Model file for the job. Use its own axes, mm. A direction names the side the tool comes from. Coordinates: 2 decimals unless noted, no trailing zeros. Order: outer loops, then holes, each group sorted by start corner. A loop starts at its lowest first (then second) coordinate and runs counter-clockwise, first axis right, second up. Notation, with made-up numbers: (19, 87.5) -> (45, 87.5) arc R20 cw to (45, 106.5) -> close; hole circle Ø3 at (79, 74.5). An arc over 180 degrees is marked (long way). Use CSV: the item, a comma, the result in double quotes. Start each with the question number.
(1) Cut at A-A on x = 18. Write the cut outline in (y, z), plus the area to 3 significant figures.
(2) Cut at B-B on y = 58.25. Write the cut outline in (x, z).
(3) Probe L1, parallel to Y at x = 18, z = 0.65; L2, parallel to X at y = 58, z = 2.05; L3, parallel to X at y = 43, z = 2.05. List the from-to ranges inside material, lowest first.
(4) Tool access for faces 4 (the flat face through (-22, 55, 1)), 5 (the flat face through (38, 33, 1)), 6 (the flat face through (1, 0, 1)): list every direction of +Z, -Z, +X, -X, +Y, -Y with a clear straight run to the whole face (end or side of a thin tool).
(5) Cut at D-D on x = -26. Write the cut outline in (y, z).
(6) Pin check, flat tips, straight feed: pin 1 Ø3 at (x, y) = (-18, 41.75) entering from -Z (3 decimals); pin 2 Ø1.5 at (x, z) = (38, 2) entering from +Y; pin 3 Ø1.5 at (y, z) = (58.5, 1) entering from +X. Stop position of each tip, or through.
(7) Cut at C-C on z = 2.4. Give the number of separate pieces and of enclosed holes in the cut face, plus the area to 3 significant figures.
(8) Pull direction Y, two halves, no side cores. Call faces 1 (the flat face through (40, 17, 1)), 2 (the cylindrical face through (26.51, 37.28, 1.52)), 3 (the cylindrical face through (17.566, 39.798, 1.521)): pulls with the +Y half, pulls with the -Y half, needs draft (parallel to the pull), parting line crosses it, or undercut.
```python
from build123d import *

# Parameters (mm, degrees)
EXTRUDE_1_DEPTH     = 3
SKETCH_2_R          = 2
CUT_EXTRUDE_1_DEPTH = 75.054456314
SKETCH_3_R          = 1.5
CUT_EXTRUDE_2_DEPTH = 75.054456314
FILLET_1_R          = 15


with BuildPart() as part:
    # 草图1 → 凸台-拉伸1 (new body)
    with BuildSketch(Plane.XY):
        Polygon((40, 0), (-40, 0), (-40, 33), (-22, 33), (-22, 62.25), (22, 62.25), (22, 33), (40, 33), align=None)
    extrude(amount=EXTRUDE_1_DEPTH)

    # 草图2 → 切除-拉伸1 (cut, through all)
    with BuildSketch(Plane.XY.offset(3)):
        with Locations((-18, 58.25)):
            Circle(SKETCH_2_R)
        with Locations((-18, 41.75)):
            Circle(SKETCH_2_R)
        with Locations((18, 41.75)):
            Circle(SKETCH_2_R)
        with Locations((18, 58.25)):
            Circle(SKETCH_2_R)
    extrude(amount=-CUT_EXTRUDE_1_DEPTH, mode=Mode.SUBTRACT)

    # 草图3 → 切除-拉伸2 (cut, through all)
    with BuildSketch(Plane.XY.offset(3)):
        with Locations((-22, 28.125)):
            Circle(SKETCH_3_R)
        with Locations((22, 28.125)):
            Circle(SKETCH_3_R)
        with Locations((22, 5.125)):
            Circle(SKETCH_3_R)
        with Locations((-22, 5.125)):
            Circle(SKETCH_3_R)
    extrude(amount=-CUT_EXTRUDE_2_DEPTH, mode=Mode.SUBTRACT)

    # 圆角1
    fillet_1_edges = [part.edges().sort_by_distance(p)[0] for p in [
        (-22, 33, 1.5),
        (22, 33, 1.5),
    ]]
    fillet(fillet_1_edges, radius=FILLET_1_R)


solid = part.part
```
Outcome:
1,outline,"(0, 0) -> (39.75, 0) -> (39.75, 3) -> (0, 3) -> close; (43.75, 0) -> (56.25, 0) -> (56.25, 3) -> (43.75, 3) -> close; (60.25, 0) -> (62.25, 0) -> (62.25, 3) -> (60.25, 3) -> close"
1,area,"163 mm2"
2,outline,"(-22, 0) -> (-20, 0) -> (-20, 3) -> (-22, 3) -> close; (-16, 0) -> (16, 0) -> (16, 3) -> (-16, 3) -> close; (20, 0) -> (22, 0) -> (22, 3) -> (20, 3) -> close"
3,L1,"0 to 39.75, 43.75 to 56.25, 60.25 to 62.25"
3,L2,"-22 to -19.98, -16.02 to 16.02, 19.98 to 22"
3,L3,"-22.86 to -19.56, -16.44 to 16.44, 19.56 to 22.86"
4,face 4,"+Z, -Z, -X, +Y"
4,face 5,"+Z, -Z, +X, +Y"
4,face 6,"+Z, -Z, +X, -X, -Y"
5,outline,"(0, 0) -> (37.8, 0) -> (37.8, 3) -> (0, 3) -> close"
6,pin 1,"through"
6,pin 2,"y = 33"
6,pin 3,"x = 22"
7,separate pieces,"1"
7,enclosed holes,"8"
7,area,"3,950 mm2"
8,face 1,"needs draft"
8,face 2,"pulls with the +Y half"
8,face 3,"undercut"
